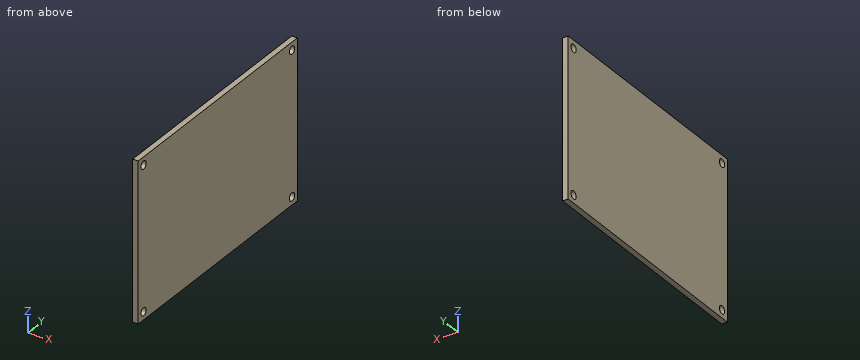
from build123d import *

# Parameters (mm, degrees)
SKETCH_R      = 1
EXTRUDE_DEPTH = 1.4
BOX001_W      = 1.4
BOX001_H      = 60
BOX001_DEPTH  = 40


with BuildPart() as extrude_body:
    # Sketch (on Face2 of Box001) → Extrude (new body)
    with BuildSketch(Plane.YZ.offset(1.4)):
        with Locations((2, 38)):
            Circle(SKETCH_R)
        with Locations((58, 38)):
            Circle(SKETCH_R)
        with Locations((58, 2)):
            Circle(SKETCH_R)
        with Locations((2, 2)):
            Circle(SKETCH_R)
    extrude(amount=-EXTRUDE_DEPTH)


with BuildPart() as board002:
    # Box001 → Box001 (new body)
    with BuildSketch(Plane.XY):
        with Locations((0.7, 30)):
            Rectangle(BOX001_W, BOX001_H)
    extrude(amount=BOX001_DEPTH)

    # Cut: cut Extrude body
    add(extrude_body.part, mode=Mode.SUBTRACT)


with BuildPart() as board002_1:
    # Cut placement: moved
    add(board002.part.moved(Location((18.5, -18, -2))))


solid = board002_1.part
Geometry: final body of the model. Coordinates: model frame, mm. Round coordinates to 2 decimals unless told otherwise and drop trailing zeros. Loops run counter-clockwise (first coordinate to the right, second up) from the corner with the lowest first, then second, coordinate; pieces in that order, holes last.
Q1. Pin query (flat end, axial travel): P1, Ø2.5, axis at y = 40, z = 0, coming from the +X side. Return the tip coordinate at first contact, or that it passes through.
Q2. Section B-B on z = 36. Return loops of the section in (x, y).
Q3. Material intervals for L1, parallel to Z at x = 19.3, y = -16; L2, parallel to Y at x = 18.9, z = 0.5, sorted ascending.
Q4. Section A-A on y = 40. Return loops of the section in (x, z), plus the area to 3 significant figures.
Evaluation:
1. P1: stops at x = 19.9
2. outline: (18.5, -18) - (19.9, -18) - (19.9, -17) - (18.5, -17) - close; (18.5, -15) - (19.9, -15) - (19.9, 39) - (18.5, 39) - close; (18.5, 41) - (19.9, 41) - (19.9, 42) - (18.5, 42) - close
3. L1: z = -2 to -1, 1 to 35, 37 to 38
3. L2: y = -18 to -16.87, -15.13 to 39.13, 40.87 to 42
4. outline: (18.5, -2) - (19.9, -2) - (19.9, -1) - (18.5, -1) - close; (18.5, 1) - (19.9, 1) - (19.9, 35) - (18.5, 35) - close; (18.5, 37) - (19.9, 37) - (19.9, 38) - (18.5, 38) - close
4. area: 50.4 mm2
